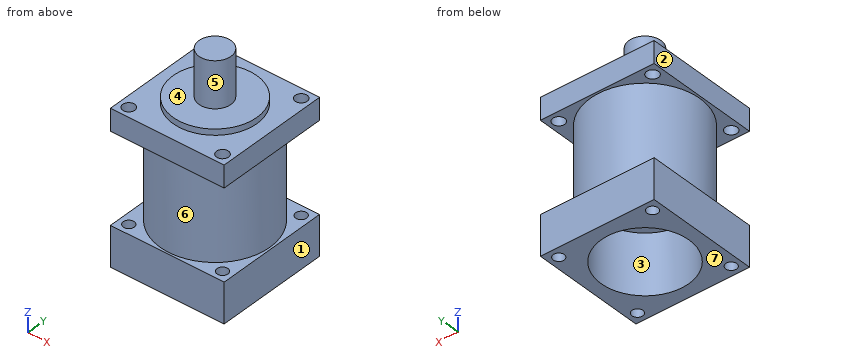
```python
from build123d import *

# Parameters (mm, degrees)
SKETCH_1_W          = 57
SKETCH_1_H          = 57
SKETCH_1_R          = 3.010136902
EXTRUDE_1_DEPTH     = 11
SKETCH_2_R          = 21
EXTRUDE_2_DEPTH     = 3
SKETCH_3_R          = 8
EXTRUDE_3_DEPTH     = 23
SKETCH_4_R          = 27.5
EXTRUDE_4_DEPTH     = 45
SKETCH_5_W          = 57
SKETCH_5_H          = 57
EXTRUDE_5_DEPTH     = 20
SKETCH_6_R          = 2.75
CUT_EXTRUDE_1_DEPTH = 115.656991337
SKETCH_7_R          = 22.011376544
CUT_EXTRUDE_2_DEPTH = 30


with BuildPart() as part:
    # 草图1 → 凸台-拉伸1 (new body)
    with BuildSketch(Plane.XY):
        with Locations((4.996753247, 11.751623377)):
            Rectangle(SKETCH_1_W, SKETCH_1_H)
        with Locations((-18.503246753, 35.251623377)):
            Circle(SKETCH_1_R, mode=Mode.SUBTRACT)
        with Locations(Location((28.496753247, 35.251623377, 0), (0, 0, 180))):
            Circle(SKETCH_1_R, mode=Mode.SUBTRACT)
        with Locations(Location((-18.503246753, -11.748376623, 0), (0, 0, 180))):
            Circle(SKETCH_1_R, mode=Mode.SUBTRACT)
        with Locations((28.496753247, -11.748376623)):
            Circle(SKETCH_1_R, mode=Mode.SUBTRACT)
    extrude(amount=EXTRUDE_1_DEPTH)

    # 草图2 → 凸台-拉伸2 (add)
    with BuildSketch(Plane.XY.offset(11)):
        with Locations((4.996753247, 11.751623377)):
            Circle(SKETCH_2_R)
    extrude(amount=EXTRUDE_2_DEPTH)

    # 草图3 → 凸台-拉伸3 (add)
    with BuildSketch(Plane.XY.offset(14)):
        with Locations((4.996753247, 11.751623377)):
            Circle(SKETCH_3_R)
    extrude(amount=EXTRUDE_3_DEPTH)

    # 草图4 → 凸台-拉伸4 (add)
    with BuildSketch(Plane(origin=(0, 0, 0), x_dir=(-1, 0, 0), z_dir=(0, 0, -1))):
        with Locations(Location((-4.996753247, 11.751623377, 0), (0, 0, 180))):
            Circle(SKETCH_4_R)
    extrude(amount=EXTRUDE_4_DEPTH)

    # 草图5 → 凸台-拉伸5 (add)
    with BuildSketch(Plane(origin=(0, 0, -45), x_dir=(-1, 0, 0), z_dir=(0, 0, -1))):
        with Locations((-4.996753247, 11.751623377)):
            Rectangle(SKETCH_5_W, SKETCH_5_H)
    extrude(amount=EXTRUDE_5_DEPTH)

    # 草图6 → 切除-拉伸1 (cut, through all)
    with BuildSketch(Plane(origin=(0, 0, -65), x_dir=(-1, 0, 0), z_dir=(0, 0, -1))):
        with Locations((-28.496753247, 35.251623377)):
            Circle(SKETCH_6_R)
        with Locations(Location((18.503246753, 35.251623377, 0), (0, 0, 180))):
            Circle(SKETCH_6_R)
        with Locations(Location((18.503246753, -11.748376623, 0), (0, 0, 180))):
            Circle(SKETCH_6_R)
        with Locations((-28.496753247, -11.748376623)):
            Circle(SKETCH_6_R)
    extrude(amount=-CUT_EXTRUDE_1_DEPTH, mode=Mode.SUBTRACT)

    # 草图7 → 切除-拉伸2 (cut)
    with BuildSketch(Plane(origin=(0, 0, -65), x_dir=(-1, 0, 0), z_dir=(0, 0, -1))):
        with Locations((-4.996753247, 11.751623377)):
            Circle(SKETCH_7_R)
    extrude(amount=-CUT_EXTRUDE_2_DEPTH, mode=Mode.SUBTRACT)


solid = part.part
```
Read the model definition and answer for the solid it produces. Units are mm, in the model's axes. Face numbers are marked on the shaded views. A direction names the side the tool comes from. Give positions to 0.01 mm unless a question says otherwise; leave off trailing zeros. Order: outer loops, then holes, each group sorted by start corner. A loop starts at its lowest first (then second) coordinate and runs counter-clockwise, first axis right, second up.
(1) Straight lines are drawn through the part: L1, parallel to Z at x = -21, y = 28; L2, parallel to Z at x = 4, y = -13; L3, parallel to Z at x = 12.5, y = 17.5. For each, find the intervals that lie inside material, in ascending order.
(2) Find section D-D (x = 16). Give the vertices of the cut face in (y, z), plus the area to 3 significant figures.
(3) Given pin 1 (2 mm diameter, centred on x = 27, y = 21, fed in from +Z); pin 2 (5 mm diameter, centred on y = 15.5, z = -21.5, fed in from -X); pin 3 (8 mm diameter, centred on x = 15, y = 28.5, fed in from +Z); pin 4 (5 mm diameter, centred on x = 28.5, y = -11.75, fed in from +Z), each flat-ended and moving along its own axis, determine where each tip first touches the part or whether it passes through.
(4) For the marked faces 5, 6 and 7, determine the directions among +Z, -Z, +X, -X, +Y, -Y from which every point of the face is accessible in a straight line to the end or side of a thin tool.
(5) Find section C-C (y = 9). Give the vertices of the cut face in (x, z), plus the area to 3 significant figures.
(6) Find section B-B (z = -49). Give the vertices of the cut face in (x, y), plus the area to 3 significant figures.
(7) For a pull along X with two mould halves and no side action, classify the marked faces 1, 2, 3 and 4 as released by +X, released by -X, zero draft, split by the parting line, or undercut.
(8) Find section A-A (x = -19). Give the vertices of the cut face in (y, z).
Result sheet:
1. L1: z = -65 to -45, 0 to 11
1. L2: z = -65 to 11
1. L3: z = -35 to 14
2. outline: (-16.75, -65) - (-7.31, -65) - (-7.31, -35) - (30.82, -35) - (30.82, -65) - (40.25, -65) - (40.25, -45) - (36.95, -45) - (36.95, 0) - (40.25, 0) - (40.25, 11) - (29.64, 11) - (29.64, 14) - (-6.13, 14) - (-6.13, 11) - (-16.75, 11) - (-16.75, 0) - (-13.45, 0) - (-13.45, -45) - (-16.75, -45) - close
2. area: 3,000 mm2
3. pin 1: stops at z = 11
3. pin 2: stops at x = -22.47
3. pin 3: stops at z = 14
3. pin 4: passes through
4. face 5: +Z
4. face 6: none
4. face 7: -Z, +X, -X, +Y, -Y
5. outline: (-23.5, -65) - (-16.84, -65) - (-16.84, -35) - (26.84, -35) - (26.84, -65) - (33.5, -65) - (33.5, -45) - (32.36, -45) - (32.36, 0) - (33.5, 0) - (33.5, 11) - (25.82, 11) - (25.82, 14) - (12.51, 14) - (12.51, 37) - (-2.52, 37) - (-2.52, 14) - (-15.82, 14) - (-15.82, 11) - (-23.5, 11) - (-23.5, 0) - (-22.37, 0) - (-22.37, -45) - (-23.5, -45) - close
5. area: 3,390 mm2
6. outline: (-23.5, -16.75) - (33.5, -16.75) - (33.5, 40.25) - (-23.5, 40.25) - close; hole circle Ø5.5 at (-18.5, -11.75); hole circle Ø5.5 at (-18.5, 35.25); hole circle Ø44.02 at (5, 11.75); hole circle Ø5.5 at (28.5, -11.75); hole circle Ø5.5 at (28.5, 35.25)
6. area: 1,630 mm2
7. face 1: released by +X
7. face 2: released by -X
7. face 3: undercut
7. face 4: zero draft
8. outline: (-16.75, -65) - (-14.45, -65) - (-14.45, -45) - (-16.75, -45) - close; (-16.75, 0) - (-14.72, 0) - (-14.72, 11) - (-16.75, 11) - close; (-9.04, -65) - (32.55, -65) - (32.55, -45) - (25.18, -45) - (25.18, 0) - (32.28, 0) - (32.28, 11) - (-8.78, 11) - (-8.78, 0) - (-1.68, 0) - (-1.68, -45) - (-9.04, -45) - close; (37.96, -65) - (40.25, -65) - (40.25, -45) - (37.96, -45) - close; (38.22, 0) - (40.25, 0) - (40.25, 11) - (38.22, 11) - close
